Answer from the drawing. Dimensions are ordinates in mm from the lowest x, y and z of the part. A direction names the side the tool comes from. Coordinates: 2 decimals unless noted, no trailing zeros. Write each loop counter-clockwise with the first axis right and the second up, starting at its lowest first coordinate (ties: lowest second). Pieces come first, ordered by that corner, then holes.
(1) The part is cut by section A-A, the plane x = 3.5. Determine the outline of the cut face in (y, z), and give its area (3 significant figures).
(2) The part is cut by section D-D, the plane z = 4. Determine the outline of the cut face in (x, y) (1 decimal).
(3) Determine the mould class of the marked faces 1, 2, 3 and 4 for opening direction Z: pulls with the +Z half, pulls with the -Z half, needs draft (parallel to the pull), parting line crosses it, or undercut.
(4) The part is cut by section B-B, the plane y = 28.8. Determine the outline of the cut face in (x, z) (1 decimal).
(5) Straight lines are drawn through the part: line 1 along X through (y, z) = (4.75, 7); line 2 along Y through (x, z) = (27.75, 7); line 3 along Z through (x, y) = (37, 1). For each, find the intervals that lie inside material, in ascending order.
(6) The part is cut by section C-C, the plane y = 20. Determine the outline of the cut face in (x, z), and give its area (3 significant figures).
(7) Given pin 1 (1.5 mm diameter, centred on y = 14.5, z = 3, fed in from -X); pin 2 (5 mm diameter, centred on y = 9.5, z = 5, fed in from +X); pin 3 (5 mm diameter, centred on x = 7.5, z = 3.5, fed in from +Y), each flat-ended and moving along its own axis, determine where each tip first touches the part or whether it passes through.
(8) Which of the six approach directions +Z, -Z, +X, -X, +Y, -Y give full straight-line access (tool end or side, diameter ignored) to the marked faces 5, 6 and 7?
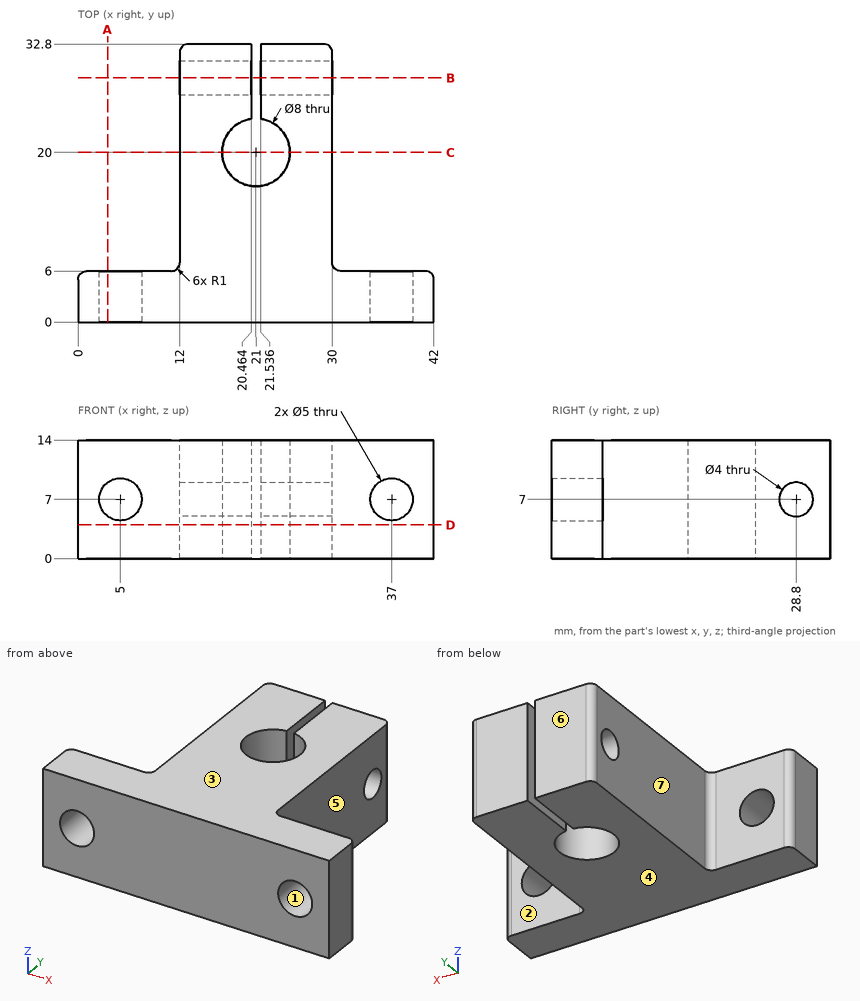
Computed:
1. outline: (0, 0) - (6, 0) - (6, 5) - (0, 5) - close; (0, 9) - (6, 9) - (6, 14) - (0, 14) - close
1. area: 60.0 mm2
2. outline: (0, 0) - (42, 0) - (42, 5) arc R1 ccw to (41, 6) - (31, 6) arc R1 cw to (30, 7) - (30, 31.8) arc R1 ccw to (29, 32.8) - (21.5, 32.8) - (21.5, 24) arc R4 cw (long way) to (20.5, 24) - (20.5, 32.8) - (13, 32.8) arc R1 ccw to (12, 31.8) - (12, 7) arc R1 cw to (11, 6) - (1, 6) arc R1 ccw to (0, 5) - close
3. face 1: undercut
3. face 2: needs draft
3. face 3: pulls with the +Z half
3. face 4: pulls with the -Z half
4. outline: (12, 0) - (20.5, 0) - (20.5, 5) - (12, 5) - close; (12, 9) - (20.5, 9) - (20.5, 14) - (12, 14) - close; (21.5, 0) - (30, 0) - (30, 5) - (21.5, 5) - close; (21.5, 9) - (30, 9) - (30, 14) - (21.5, 14) - close
5. line 1: x = 0 to 2.5, 7.5 to 34.5, 39.5 to 42
5. line 2: y = 0 to 26.8, 30.8 to 32.8
5. line 3: z = 0 to 4.5, 9.5 to 14
6. outline: (12, 0) - (17, 0) - (17, 14) - (12, 14) - close; (25, 0) - (30, 0) - (30, 14) - (25, 14) - close
6. area: 140 mm2
7. pin 1: stops at x = 12
7. pin 2: stops at x = 30
7. pin 3: stops at y = 6
8. face 5: +Z, -Z, +X, +Y
8. face 6: +Z, -Z, +X, -X, +Y
8. face 7: +Z, -Z, -X, +Y
